```python
from build123d import *

# Parameters (mm, degrees)
BOSS_EXTRUDE1_DEPTH = 50
CUT_EXTRUDE1_DEPTH  = 47
CHAMFER3_SIZE       = 3
SKETCH5_W           = 56
SKETCH5_H           = 18
CUT_EXTRUDE2_DEPTH  = 3
SKETCH6_W           = 85
SKETCH6_H           = 18
CUT_EXTRUDE3_DEPTH  = 3
SKETCH7_W           = 50
SKETCH7_H           = 20
CUT_EXTRUDE4_DEPTH  = 3
SKETCH8_W           = 44
SKETCH8_H           = 20
CUT_EXTRUDE5_DEPTH  = 3
SKETCH9_W           = 11
SKETCH9_H           = 2
CUT_EXTRUDE6_DEPTH  = 1
DRAFT3_START        = -46.843617021
DRAFT3_DEPTH        = 11
SKETCH12_W          = 11
SKETCH12_H          = 2
CUT_EXTRUDE7_DEPTH  = 1
DRAFT4_START        = -46.843617021
DRAFT4_DEPTH        = 11


# Read off the part's stored shape, not the designer's step: Draft3, Draft4
with BuildPart() as part:
    # Sketch1 → Boss-Extrude1 (new body)
    with BuildSketch(Plane(origin=(0, 0, 0), x_dir=(1, 0, 0), z_dir=(0, 1, 0))):
        Polygon((-88.764893617, 6.343617021), (115.235106383, 6.343617021), (115.235106383, 76.343617021), (65.235106383, 76.343617021), (65.235106383, 126.343617021), (-38.764893617, 126.343617021), (-38.764893617, 76.343617021), (-88.764893617, 76.343617021), align=None)
    extrude(amount=BOSS_EXTRUDE1_DEPTH)

    # Sketch4 → Cut-Extrude1 (cut)
    with BuildSketch(Plane(origin=(0, 50, 0), x_dir=(1, 0, 0), z_dir=(0, 1, 0))):
        Polygon((-35.764893617, 123.343617021), (-35.764893617, 73.343617021), (-85.764893617, 73.343617021), (-85.764893617, 9.343617021), (112.235106383, 9.343617021), (112.235106383, 73.343617021), (62.235106383, 73.343617021), (62.235106383, 123.343617021), align=None)
    extrude(amount=-CUT_EXTRUDE1_DEPTH, mode=Mode.SUBTRACT)

    # Chamfer3
    chamfer3_edges = [part.edges().sort_by_distance(p)[0] for p in [
        (13.235106383, 50, -123.343617021),
        (-35.764893617, 50, -98.343617021),
        (-60.764893617, 50, -73.343617021),
        (-85.764893617, 50, -41.343617021),
        (13.235106383, 50, -9.343617021),
        (112.235106383, 50, -41.343617021),
        (87.235106383, 50, -73.343617021),
        (62.235106383, 50, -98.343617021),
    ]]
    chamfer(chamfer3_edges, length=CHAMFER3_SIZE - 0.0001)  # a hair under: the kernel refuses the full size

    # Sketch5 → Cut-Extrude2 (cut)
    with BuildSketch(Plane(origin=(115.235106383, 0, 0), x_dir=(0, 0, -1), z_dir=(1, 0, 0))):
        with Locations((37.343617021, 17)):
            Rectangle(SKETCH5_W, SKETCH5_H)
    extrude(amount=-CUT_EXTRUDE2_DEPTH, mode=Mode.SUBTRACT)

    # Sketch6 → Cut-Extrude3 (cut)
    with BuildSketch(Plane.XY.offset(-6.343617021)):
        with Locations((69.735106383, 17)):
            Rectangle(SKETCH6_W, SKETCH6_H)
    extrude(amount=-CUT_EXTRUDE3_DEPTH, mode=Mode.SUBTRACT)

    # Sketch7 → Cut-Extrude4 (cut)
    with BuildSketch(Plane.ZY.offset(88.764893617)):
        with Locations((-41.343617021, 18)):
            Rectangle(SKETCH7_W, SKETCH7_H)
    extrude(amount=-CUT_EXTRUDE4_DEPTH, mode=Mode.SUBTRACT)

    # Sketch8 → Cut-Extrude5 (cut)
    with BuildSketch(Plane(origin=(0, 0, -126.343617021), x_dir=(-1, 0, 0), z_dir=(0, 0, -1))):
        with Locations((-13.235106383, 25)):
            Rectangle(SKETCH8_W, SKETCH8_H)
    extrude(amount=-CUT_EXTRUDE5_DEPTH, mode=Mode.SUBTRACT)

    # Sketch9 → Cut-Extrude6 (cut)
    with BuildSketch(Plane(origin=(115.235106383, 0, 0), x_dir=(0, 0, -1), z_dir=(1, 0, 0))):
        with Locations((41.343617021, 41)):
            Rectangle(SKETCH9_W, SKETCH9_H)
    extrude(amount=-CUT_EXTRUDE6_DEPTH, mode=Mode.SUBTRACT)

    # Draft3 outline → Draft3 (add)
    with BuildSketch(Plane.XY.offset(DRAFT3_START)):
        Polygon((114.235106383, 42), (114.235106383, 41), (115.235106383, 42), align=None)
        Polygon((115.235106383, 40), (114.235106383, 41), (114.235106383, 40), align=None)
    extrude(amount=DRAFT3_DEPTH)

    # Sketch12 → Cut-Extrude7 (cut)
    with BuildSketch(Plane.ZY.offset(88.764893617)):
        with Locations((-41.343617021, 41)):
            Rectangle(SKETCH12_W, SKETCH12_H)
    extrude(amount=-CUT_EXTRUDE7_DEPTH, mode=Mode.SUBTRACT)

    # Draft4 outline → Draft4 (add)
    with BuildSketch(Plane.XY.offset(DRAFT4_START)):
        Polygon((-87.764893617, 42), (-88.764893617, 42), (-87.764893617, 41), align=None)
        Polygon((-87.764893617, 40), (-87.764893617, 41), (-88.764893617, 40), align=None)
    extrude(amount=DRAFT4_DEPTH)


solid = part.part
```
Geometry: final body of the model. Coordinates: model frame, mm. A direction names the side the tool comes from. Coordinates: 2 decimals unless noted, no trailing zeros. Order: outer loops, then holes, each group sorted by start corner. A loop starts at its lowest first (then second) coordinate and runs counter-clockwise, first axis right, second up. Notation, with made-up numbers: (-27, 44) -> (27, 44) arc R23 ccw to (27, 82) -> close; hole circle Ø7 at (24.25, 34.5). An arc over 180 degrees is marked (long way). Use CSV: the item, a comma, the result in double quotes.
1) Access query for faces 1 (the flat face through (-63, 25, -76.344)), 2 (the flat face through (14, 14, -126.344)), 3 (the flat face through (91, 25, -76.344)), 4 (the flat face through (-35.765, 25, -99)). Directions: +Z, -Z, +X, -X, +Y, -Y. A direction counts if a zero-diameter tool reaches every point of the face in a straight line with its end or side. Return the directions, or none.
Findings:
face 1,"-Z, -X, +Y, -Y"
face 2,"-Z, +X, -X, +Y, -Y"
face 3,"-Z, +X, +Y, -Y"
face 4,"+Y"
2) Section B-B on z = -53.5. State how many separate pieces and enclosed holes the cut face has, then the cut area to 3 significant figures.
Findings:
separate pieces,"3"
enclosed holes,"0"
area,"771 mm^2"
3) Section D-D on y = 11. Output: boundary loops of the cut face in (x, z), then the cut area to 4 significant figures.
Findings:
outline,"(-88.76, -76.34) -> (-38.76, -76.34) -> (-38.76, -126.34) -> (65.24, -126.34) -> (65.24, -76.34) -> (115.24, -76.34) -> (115.24, -65.34) -> (112.24, -65.34) -> (112.24, -73.34) -> (62.24, -73.34) -> (62.24, -123.34) -> (-35.76, -123.34) -> (-35.76, -73.34) -> (-85.76, -73.34) -> (-85.76, -66.34) -> (-88.76, -66.34) -> close; (-88.76, -16.34) -> (-85.76, -16.34) -> (-85.76, -9.34) -> (27.24, -9.34) -> (27.24, -6.34) -> (-88.76, -6.34) -> close; (112.24, -9.34) -> (115.24, -9.34) -> (115.24, -6.34) -> (112.24, -6.34) -> close"
area,"1,335 mm^2"
4) Line query: line 1 (Z direction, x = -75.5, y = 20.5); line 2 (X direction, y = 47, z = -48); line 3 (Z direction, x = 2.5, y = 7). Output: solid intervals per line, ascending.
Findings:
line 1,"z = -76.34 to -73.34, -9.34 to -6.34"
line 2,"x = -88.76 to -85.76, 112.24 to 115.24"
line 3,"z = -126.34 to -123.34, -9.34 to -6.34"
5) Pin query (flat end, axial travel): pin 1 Ø1.5 at (y, z) = (41, -85.5) entering from -X; pin 2 Ø22 at (y, z) = (31, -97) entering from +X; pin 3 Ø1.5 at (x, y) = (-87.5, 19.5) entering from -Z. Return the tip coordinate at first contact, or that it passes through.
Findings:
pin 1,"stops at x = -38.76"
pin 2,"stops at x = 65.24"
pin 3,"stops at z = -76.34"
6) Mould query, pull axis X, two halves, no side actions, for faces 5 (the flat face through (-85.765, 30, -42)), 6 (the flat face through (-88.765, 30, -42)), 7 (the flat face through (12, 0, -54)). Classes: +X half, -X half, draft (parallel to the pull), parting line (faces both ways), or undercut.
Findings:
face 5,"undercut"
face 6,"-X half"
face 7,"draft"
